Can you work these out from the model? Positions are in its coordinate system, mm. A direction names the side the tool comes from. Give positions to 0.01 mm unless a question says otherwise; leave off trailing zeros. Write item = value, one per line.
from build123d import *

# Parameters (mm, degrees)
SKETCH3_R            = 27.94
BOSS_EXTRUDE2_DEPTH  = 122.46
SKETCH5_R            = 3.175
CUT_EXTRUDE1_DEPTH   = 129.676877488
SKETCH4_W            = 14
SKETCH4_H            = 6
SHELL1_START         = 3
SHELL1_OUTLINE_R     = 10.94
SHELL1_OUTLINE_R_2   = 6.175
SHELL1_DEPTH         = 116.46
SHELL1_2_OUTLINE_R   = 24.94
SHELL1_2_OUTLINE_R_2 = 10.94
SHELL1_2_DEPTH       = 10.72
SHELL1_START_2       = 109.72
SHELL1_3_OUTLINE_R   = 24.94
SHELL1_3_OUTLINE_R_2 = 10.94
SHELL1_3_DEPTH       = 9.74
SHELL1_START_3       = 25.72
SHELL1_4_OUTLINE_R   = 24.94
SHELL1_4_OUTLINE_R_2 = 10.94
SHELL1_4_DEPTH       = 9
SHELL1_START_4       = 46.72
SHELL1_5_OUTLINE_R   = 24.94
SHELL1_5_OUTLINE_R_2 = 10.94
SHELL1_5_DEPTH       = 9
SHELL1_START_5       = 67.72
SHELL1_6_OUTLINE_R   = 24.94
SHELL1_6_OUTLINE_R_2 = 10.94
SHELL1_6_DEPTH       = 9
SHELL1_START_6       = 88.72
SHELL1_7_OUTLINE_R   = 24.94
SHELL1_7_OUTLINE_R_2 = 10.94
SHELL1_7_DEPTH       = 9
BOSS_EXTRUDE3_REACH  = 130.677
SKETCH13_W           = 16.483162312
SKETCH13_H           = 6
CUT_EXTRUDE3_DEPTH   = 123


# Read off the part's stored shape, not the designer's step: Shell1
with BuildPart() as part:
    # Sketch3 → Boss-Extrude2 (new body)
    with BuildSketch(Plane.XY):
        Circle(SKETCH3_R)
    extrude(amount=BOSS_EXTRUDE2_DEPTH)

    # Sketch5 → Cut-Extrude1 (cut, through all)
    with BuildSketch(Plane.XY.offset(122.46)):
        Circle(SKETCH5_R)
    extrude(amount=-CUT_EXTRUDE1_DEPTH, mode=Mode.SUBTRACT)

    # Sketch4 → Cut-Revolve1 (revolve, cut)
    with BuildSketch(Plane(origin=(0, 0, 0), x_dir=(1, 0, 0), z_dir=(0, 1, 0)), mode=Mode.PRIVATE) as cut_revolve1_sk:
        with Locations((-20.94, -103.72)):
            Rectangle(SKETCH4_W, SKETCH4_H)
        with Locations((-20.94, -82.72)):
            Rectangle(SKETCH4_W, SKETCH4_H)
        with Locations((-20.94, -61.72)):
            Rectangle(SKETCH4_W, SKETCH4_H)
        with Locations((-20.94, -40.72)):
            Rectangle(SKETCH4_W, SKETCH4_H)
        with Locations((-20.94, -19.72)):
            Rectangle(SKETCH4_W, SKETCH4_H)
    revolve(cut_revolve1_sk.sketch.rotate(Axis((0, 0, 122.46), (0, 0, -1)), 180), axis=Axis((0, 0, 122.46), (0, 0, -1)), mode=Mode.SUBTRACT)

    # Shell1 outline → Shell1 (cut)
    with BuildSketch(Plane.XY.offset(SHELL1_START)):
        Circle(SHELL1_OUTLINE_R)
        Circle(SHELL1_OUTLINE_R_2, mode=Mode.SUBTRACT)
    extrude(amount=SHELL1_DEPTH, mode=Mode.SUBTRACT)

    # Shell1 2 outline → Shell1 2 (cut)
    with BuildSketch(Plane.XY.offset(SHELL1_START)):
        Circle(SHELL1_2_OUTLINE_R)
        Circle(SHELL1_2_OUTLINE_R_2, mode=Mode.SUBTRACT)
    extrude(amount=SHELL1_2_DEPTH, mode=Mode.SUBTRACT)

    # Shell1 3 outline → Shell1 3 (cut)
    with BuildSketch(Plane.XY.offset(SHELL1_START_2)):
        Circle(SHELL1_3_OUTLINE_R)
        Circle(SHELL1_3_OUTLINE_R_2, mode=Mode.SUBTRACT)
    extrude(amount=SHELL1_3_DEPTH, mode=Mode.SUBTRACT)

    # Shell1 4 outline → Shell1 4 (cut)
    with BuildSketch(Plane.XY.offset(SHELL1_START_3)):
        Circle(SHELL1_4_OUTLINE_R)
        Circle(SHELL1_4_OUTLINE_R_2, mode=Mode.SUBTRACT)
    extrude(amount=SHELL1_4_DEPTH, mode=Mode.SUBTRACT)

    # Shell1 5 outline → Shell1 5 (cut)
    with BuildSketch(Plane.XY.offset(SHELL1_START_4)):
        Circle(SHELL1_5_OUTLINE_R)
        Circle(SHELL1_5_OUTLINE_R_2, mode=Mode.SUBTRACT)
    extrude(amount=SHELL1_5_DEPTH, mode=Mode.SUBTRACT)

    # Shell1 6 outline → Shell1 6 (cut)
    with BuildSketch(Plane.XY.offset(SHELL1_START_5)):
        Circle(SHELL1_6_OUTLINE_R)
        Circle(SHELL1_6_OUTLINE_R_2, mode=Mode.SUBTRACT)
    extrude(amount=SHELL1_6_DEPTH, mode=Mode.SUBTRACT)

    # Shell1 7 outline → Shell1 7 (cut)
    with BuildSketch(Plane.XY.offset(SHELL1_START_6)):
        Circle(SHELL1_7_OUTLINE_R)
        Circle(SHELL1_7_OUTLINE_R_2, mode=Mode.SUBTRACT)
    extrude(amount=SHELL1_7_DEPTH, mode=Mode.SUBTRACT)

    # Boss-Extrude3: up to this face of the body (flat: up to its plane)
    boss_extrude3_end = Plane(part.part.faces().sort_by_distance((-27.149737461, 0, 122.46))[0])
    # Sketch10 → Boss-Extrude3 (add, up to the picked face)
    with BuildSketch(Plane(origin=(0, 0, 0), x_dir=(-1, 0, 0), z_dir=(0, 0, -1)), mode=Mode.PRIVATE) as boss_extrude3_sk1:
        with BuildLine():
            Line((-1, 27.922098775), (-1, 3.01340754))
            ThreePointArc((-1, 3.01340754), (0, 3.175), (1, 3.01340754))
            Line((1, 3.01340754), (1, 27.922098775))
            ThreePointArc((1, 27.922098775), (0, 27.94), (-1, 27.922098775))
        make_face()
    boss_extrude3_tool1 = split(extrude(boss_extrude3_sk1.sketch, amount=-BOSS_EXTRUDE3_REACH, mode=Mode.PRIVATE), bisect_by=boss_extrude3_end, keep=Keep.BOTH, mode=Mode.PRIVATE)
    # Sketch10 → Boss-Extrude3 (add, up to the picked face)
    with BuildSketch(Plane(origin=(0, 0, 0), x_dir=(-1, 0, 0), z_dir=(0, 0, -1)), mode=Mode.PRIVATE) as boss_extrude3_sk2:
        with BuildLine():
            Line((3.01340754, 1), (27.922098775, 1))
            ThreePointArc((27.922098775, 1), (27.94, 0), (27.922098775, -1))
            Line((27.922098775, -1), (3.01340754, -1))
            ThreePointArc((3.01340754, -1), (3.175, 0), (3.01340754, 1))
        make_face()
    boss_extrude3_tool2 = split(extrude(boss_extrude3_sk2.sketch, amount=-BOSS_EXTRUDE3_REACH, mode=Mode.PRIVATE), bisect_by=boss_extrude3_end, keep=Keep.BOTH, mode=Mode.PRIVATE)
    # Sketch10 → Boss-Extrude3 (add, up to the picked face)
    with BuildSketch(Plane(origin=(0, 0, 0), x_dir=(-1, 0, 0), z_dir=(0, 0, -1)), mode=Mode.PRIVATE) as boss_extrude3_sk3:
        with BuildLine():
            Line((-1, -3.01340754), (-1, -27.922098775))
            ThreePointArc((-1, -27.922098775), (0, -27.94), (1, -27.922098775))
            Line((1, -27.922098775), (1, -3.01340754))
            ThreePointArc((1, -3.01340754), (0, -3.175), (-1, -3.01340754))
        make_face()
    boss_extrude3_tool3 = split(extrude(boss_extrude3_sk3.sketch, amount=-BOSS_EXTRUDE3_REACH, mode=Mode.PRIVATE), bisect_by=boss_extrude3_end, keep=Keep.BOTH, mode=Mode.PRIVATE)
    # Sketch10 → Boss-Extrude3 (add, up to the picked face)
    with BuildSketch(Plane(origin=(0, 0, 0), x_dir=(-1, 0, 0), z_dir=(0, 0, -1)), mode=Mode.PRIVATE) as boss_extrude3_sk4:
        with BuildLine():
            Line((-27.922098775, -1), (-3.01340754, -1))
            ThreePointArc((-3.01340754, -1), (-3.175, 0), (-3.01340754, 1))
            Line((-3.01340754, 1), (-27.922098775, 1))
            ThreePointArc((-27.922098775, 1), (-27.94, 0), (-27.922098775, -1))
        make_face()
    boss_extrude3_tool4 = split(extrude(boss_extrude3_sk4.sketch, amount=-BOSS_EXTRUDE3_REACH, mode=Mode.PRIVATE), bisect_by=boss_extrude3_end, keep=Keep.BOTH, mode=Mode.PRIVATE)
    add(boss_extrude3_tool1.solids().sort_by(Axis((0, 15.527819, 0), (0, 0, 1)))[0])
    add(boss_extrude3_tool2.solids().sort_by(Axis((-15.527819, 0, 0), (0, 0, 1)))[0])
    add(boss_extrude3_tool3.solids().sort_by(Axis((0, -15.527819, 0), (0, 0, 1)))[0])
    add(boss_extrude3_tool4.solids().sort_by(Axis((15.527819, 0, 0), (0, 0, 1)))[0])

    # Sketch13 → Cut-Revolve2 (revolve, cut)
    with BuildSketch(Plane(origin=(0, 0, 0), x_dir=(1, 0, 0), z_dir=(0, 1, 0)), mode=Mode.PRIVATE) as cut_revolve2_sk:
        with Locations((-22.145666886, -40.72)):
            Rectangle(SKETCH13_W, SKETCH13_H)
        with Locations((-22.145666886, -19.72)):
            Rectangle(SKETCH13_W, SKETCH13_H)
        with Locations((-22.145666886, -61.72)):
            Rectangle(SKETCH13_W, SKETCH13_H)
        with Locations((-22.145666886, -82.72)):
            Rectangle(SKETCH13_W, SKETCH13_H)
        with Locations((-22.145666886, -103.72)):
            Rectangle(SKETCH13_W, SKETCH13_H)
    revolve(cut_revolve2_sk.sketch.rotate(Axis((0, 0, 121.588746248), (0, 0, -1)), 180), axis=Axis((0, 0, 121.588746248), (0, 0, -1)), mode=Mode.SUBTRACT)

    # Sketch16 → Cut-Extrude3 (cut)
    with BuildSketch(Plane(origin=(0, 0, 0), x_dir=(-1, 0, 0), z_dir=(0, 0, -1))):
        with BuildLine():
            Line((-27.923120749, -0.971044624), (-6.098171639, -0.971044624))
            ThreePointArc((-6.098171639, -0.971044624), (-0.014665674, -6.174982584), (6.093490379, -1))
            Line((6.093490379, -1), (27.922098775, -1))
            ThreePointArc((27.922098775, -1), (-0.014486703, -27.939996244), (-27.923120749, -0.971044624))
        make_face()
    extrude(amount=-CUT_EXTRUDE3_DEPTH, mode=Mode.SUBTRACT)


solid = part.part
Q1. Imagine slicing it at A-A, the plane z = 9. Give the number of separate pieces and of enclosed holes in the cut face, then the cut area to 3 significant figures.
Output:
separate_pieces = 1
enclosed_holes = 3
area = 455 mm2
Q2. For pin 1 (10 mm diameter, centred on x = -10, z = 97.5, fed in from +Y); pin 2 (5 mm diameter, centred on x = -5.5, y = 4.5, fed in from -Z); pin 3 (6 mm diameter, centred on x = 16, z = 81, fed in from -Y); pin 4 (5.5 mm diameter, centred on x = 19.5, z = 65.5, fed in from +Y), each with a flat end and sliding along its axis, tell me the tip position at first contact or that it passes through.
Output:
pin_1 = 27.49
pin_2 = 0
pin_3 = -0.97
pin_4 = 22.36
Q3. Which directions (+Z, -Z, +X, -X, +Y, -Y) give clear straight access to the entire face, cutting with the end or side of a thin tool? Please do faces 5 (the cylindrical face through (17.82, 17.45, 30.16)), 6 (the flat face through (12, -0.971, 60)), 7 (the flat face through (0, 16, 100.72)).
Output:
face_5 = none
face_6 = +Z, -Z, +X, -Y
face_7 = +Y
Q4. We'd pull the mould along Y, two halves only. Please class faces 1 (the flat face through (-1, 9, 60)), 2 (the cylindrical face through (-7.66, 7.81, 19.64)), 3 (the flat face through (0, 16, 43.72)), 4 (the cylindrical face through (0.137, -6.173, 60.373)): released by +Y, released by -Y, zero draft, split by the parting line, or undercut.
Output:
face_1 = undercut
face_2 = undercut
face_3 = zero draft
face_4 = released by -Y
Q5. I need wall thicknesses on L1, parallel to X at y = 12.5, z = 29.5; L2, parallel to Y at x = 1.5, z = 101.5; L3, parallel to X at y = 10.5, z = 27.5. Which ranges of each line are inside material? Lowest first, please.
Output:
L1 = -24.99 to -21.58, -1 to 1, 21.58 to 24.99
L2 = -5.99 to -2.8, 2.8 to 5.99, 10.84 to 13.82
L3 = -25.89 to -22.62, -1 to 1, 22.62 to 25.89
